```python
from build123d import *

# Parameters (mm, degrees)
F0_W      = 8.2
F0_H      = 23
F1_DEPTH  = 9.7
F2_W      = 5.2
F2_H      = 11
F2_W_2    = 4.1
F2_H_2    = 5
F3_DEPTH  = 0.2
F3_FACE_W = 4.1
F3_FACE_H = 5
F4_DEPTH  = 10.75
F5_W      = 0.75
F5_H      = 2
F5_H_2    = 1.25
F6_DEPTH  = 4.5


with BuildPart() as f1:
    # F0 (on Front) → F1 (new body)
    with BuildSketch(Plane.XZ):
        Rectangle(F0_W, F0_H)
    extrude(amount=F1_DEPTH)

    # F2 (on face) → F3 (cut)
    with BuildSketch(Plane.YZ.offset(4.1)):
        with Locations((-5.45, 0)):
            Rectangle(F2_W, F2_H)
        with Locations((-5.45, 0)):
            Rectangle(F2_W_2, F2_H_2, mode=Mode.SUBTRACT)
    extrude(amount=-F3_DEPTH, mode=Mode.SUBTRACT)

    # F3_face (on face) → F4 (join)
    with BuildSketch(Plane(origin=(4.1, -5.45, 0), x_dir=(0, 1, 0), z_dir=(1, 0, 0))):
        Rectangle(F3_FACE_W, F3_FACE_H)
    extrude(amount=F4_DEPTH)

    # F5 (on face) → F6 (join)
    with BuildSketch(Plane(origin=(0, 0, 0), x_dir=(-1, 0, 0), z_dir=(0, 1, 0))):
        with Locations((-3.725, 10.5)):
            Rectangle(F5_W, F5_H)
        with Locations((3.725, 10.5)):
            Rectangle(F5_W, F5_H)
        with Locations((3.725, -10.5)):
            Rectangle(F5_W, F5_H)
        with Locations((-3.725, -10.5)):
            Rectangle(F5_W, F5_H)
        with Locations((-1.625, -7.375)):
            Rectangle(F5_W, F5_H_2)
        with Locations((1.625, -7.375)):
            Rectangle(F5_W, F5_H_2)
        with Locations((1.625, -4.125)):
            Rectangle(F5_W, F5_H_2)
        with Locations((-1.625, -4.125)):
            Rectangle(F5_W, F5_H_2)
        with Locations((-1.625, -0.875)):
            Rectangle(F5_W, F5_H_2)
        with Locations((1.625, -0.875)):
            Rectangle(F5_W, F5_H_2)
        with Locations((1.625, 5.875)):
            Rectangle(F5_W, F5_H_2)
        with Locations((-1.625, 5.875)):
            Rectangle(F5_W, F5_H_2)
    extrude(amount=F6_DEPTH)


solid = f1.part
```
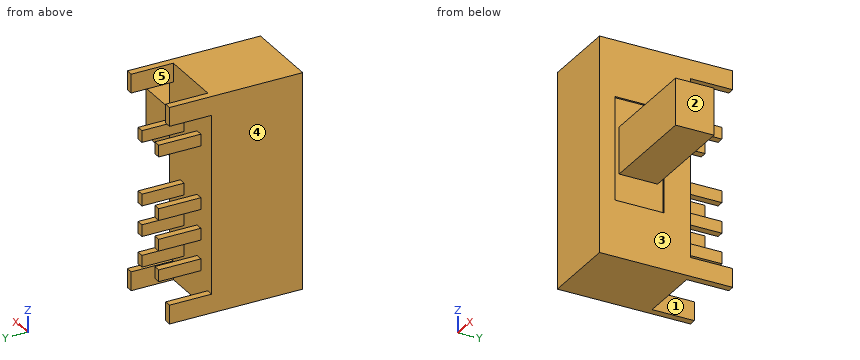
CAD build for the part. Positions are in the model's coordinates, mm. Face numbers are marked on the shaded views. A direction names the side the tool comes from. Coordinates: 2 decimals unless noted, no trailing zeros. Order: outer loops, then holes, each group sorted by start corner. A loop starts at its lowest first (then second) coordinate and runs counter-clockwise, first axis right, second up. Notation, with made-up numbers: (3, 27) - (51, 27) arc R16 ccw to (51, 48) - close; hole circle Ø7 at (39, 78.25). An arc over 180 degrees is marked (long way). Use a Markdown table: item, result. Add a question column.
(1) Saw through at D-D (x = -2.5). Give the cut face in (y, z).
(2) Flat gauge pins, fed straight in: pin 1 (5 mm diameter, centred on y = -5.5, z = 8, fed in from +X); pin 2 (2 mm diameter, centred on x = 10.5, y = -6.5, fed in from -Z); pin 3 (0.6 mm diameter, centred on x = 1.5, y = 2, fed in from -Z); pin 4 (8 mm diameter, centred on x = 9, y = 1.5, fed in from +Z). Where does each tip first touch, or does it go through?
(3) Saw through at C-C (y = 2.75). Count the separate pieces of the cut face and the enclosed holes in it, then the cut area to 3 significant figures.
(4) Pull direction X, two halves, no side cores. Call the marked faces 3, 4 and 5: +X half, -X half, draft (parallel to the pull), parting line (faces both ways), or undercut.
(5) Saw through at A-A (z = -3). Give the cut face in (x, y), then the cut area to 3 significant figures.
(6) Which spindle directions (+Z, -Z, +X, -X, +Y, -Y) get a long thin tool onto all of the face, cutting with end or side? Do the marked faces 1 and 2. Say none if no direction does.
(7) Drill centre lines: line 1 along X through (y, z) = (3, 10.25); line 2 along X through (y, z) = (1.5, -7); line 3 along X through (y, z) = (-1.75, -3.75). Where is each one in solid material? Low to high. Write a range as [from, to].
(8) Saw through at B-B (y = -4). Give the cut face in (x, z), then the cut area to 3 significant figures.
Solved:
| question | item | result |
|---|---|---|
| 1 | outline | (-9.7, -11.5) - (0, -11.5) - (0, 11.5) - (-9.7, 11.5) - close |
| 2 | pin 1 | stops at x = 4.1 |
| 2 | pin 2 | stops at z = -2.5 |
| 2 | pin 3 | stops at z = -8 |
| 2 | pin 4 | passes through |
| 3 | separate pieces | 12 |
| 3 | enclosed holes | 0 |
| 3 | area | 13.5 mm² |
| 4 | face 3 | +X half |
| 4 | face 4 | -X half |
| 4 | face 5 | undercut |
| 5 | outline | (-4.1, -9.7) - (4.1, -9.7) - (4.1, -8.05) - (3.9, -8.05) - (3.9, -2.85) - (4.1, -2.85) - (4.1, 0) - (-4.1, 0) - close |
| 5 | area | 78.5 mm² |
| 6 | face 1 | +Z, -Z, +Y |
| 6 | face 2 | +Z, -Z, +X, +Y, -Y |
| 7 | line 1 | x = [-4.1, -3.35], [3.35, 4.1] |
| 7 | line 2 | x = [-2, -1.25], [1.25, 2] |
| 7 | line 3 | x = [-4.1, 4.1] |
| 8 | outline | (-4.1, -11.5) - (4.1, -11.5) - (4.1, -5.5) - (3.9, -5.5) - (3.9, -2.5) - (14.85, -2.5) - (14.85, 2.5) - (3.9, 2.5) - (3.9, 5.5) - (4.1, 5.5) - (4.1, 11.5) - (-4.1, 11.5) - close |
| 8 | area | 241 mm² |
